from build123d import *

# Parameters (mm, degrees)
F0_W      = 38
F0_H      = 1.8
F1_DEPTH  = 50
F2_W      = 33.097349
F2_H      = 12
F2_W_2    = 36.357001
F3_DEPTH  = 25
F5_W      = 3
F5_H      = 8
F6_DEPTH  = 1.8
F10_R     = 1.2
F11_DEPTH = 43
F4_W      = 33.097349
F4_H      = 12
F4_W_2    = 36.357002
F14_DEPTH = 1


with BuildPart() as f1:
    # F0 (on Top) → F1 (new body)
    with BuildSketch(Plane.XY):
        with Locations((-19, 0)):
            Rectangle(F0_W, F0_H)
        with BuildLine():
            Line((0.167619, 0.9), (0, 0.9))
            Line((0, 0.9), (0, -0.9))
            Line((0, -0.9), (0.167619, -0.9))
            ThreePointArc((0.167619, -0.9), (5, 0), (0.167619, 0.9))
        make_face()
    extrude(amount=F1_DEPTH)

    # F2 (on Right) → F3 (cut)
    with BuildSketch(Plane.YZ):
        with Locations((2.793991, 37)):
            Rectangle(F2_W, F2_H)
        with Locations((3.725327, 13)):
            Rectangle(F2_W_2, F2_H)
    extrude(amount=F3_DEPTH, mode=Mode.SUBTRACT)

    # F5 (on face) → F6 (cut, through all)
    with BuildSketch(Plane.XZ.offset(0.9)):
        with Locations((-32.5, 25)):
            Rectangle(F5_W, F5_H)
        with Locations((-26.5, 25)):
            Rectangle(F5_W, F5_H)
        with Locations((-14.5, 25)):
            Rectangle(F5_W, F5_H)
        with Locations((-8.5, 25)):
            Rectangle(F5_W, F5_H)
    extrude(amount=-F6_DEPTH, mode=Mode.SUBTRACT)

    # F8 (on Front) → F9 (revolve)
    with BuildSketch(Plane.XZ):
        with BuildLine():
            add(Edge.make_bspline(
                [(3.7, 32.2), (3.704607, 31.503535), (3.733649, 31.405747), (4.1, 31)],
                knots=[0, 0, 0, 0, 1.264911, 1.264911, 1.264911, 1.264911], degree=3))
            Line((3.7, 32.2), (2.5, 32.2))
            Line((2.5, 32.2), (2.5, 31))
            Line((2.5, 31), (4.1, 31))
        make_face()
        with BuildLine():
            Line((2.5, 8.2), (2.5, 7))
            Line((2.5, 7), (4.2, 7))
            add(Edge.make_bspline(
                [(4.2, 7), (3.710281, 7), (3.725807, 7.664207), (3.7, 8.2)],
                knots=[0, 0, 0, 0, 1.3, 1.3, 1.3, 1.3], degree=3))
            Line((3.7, 8.2), (2.5, 8.2))
        make_face()
    revolve(axis=Axis((2.5, 0, 31.6), (0, 0, 1)))

    # F10 (on face) → F11 (join, through all)
    with BuildSketch(Plane(origin=(0, 0, 0), x_dir=(1, 0, 0), z_dir=(0, 0, -1))):
        with Locations((2.5, 0)):
            Circle(F10_R)
    extrude(amount=-F11_DEPTH)

    # F12 (on Front) → F13 (revolve)
    with BuildSketch(Plane.XZ):
        with BuildLine():
            Line((4.2, 43), (2.5, 43))
            Line((2.5, 43), (2.5, 41.8))
            Line((2.5, 41.8), (3.7, 41.8))
            add(Edge.make_bspline(
                [(4.2, 43), (3.697237, 42.880607), (3.698886, 42.436921), (3.7, 41.8)],
                knots=[0, 0, 0, 0, 1.3, 1.3, 1.3, 1.3], degree=3))
        make_face()
        with BuildLine():
            Line((4.2, 19), (2.5, 19))
            Line((2.5, 19), (2.5, 17.8))
            Line((2.5, 17.8), (3.7, 17.8))
            add(Edge.make_bspline(
                [(4.2, 19), (3.697237, 18.880607), (3.698886, 18.436921), (3.7, 17.8)],
                knots=[0, 0, 0, 0, 1.3, 1.3, 1.3, 1.3], degree=3))
        make_face()
    revolve(axis=Axis((2.5, 0, 42.4), (0, 0, -1)))

    # F4 (on Right) → F14 (cut)
    with BuildSketch(Plane.YZ):
        with Locations((-0.465668, 37)):
            Rectangle(F4_W, F4_H)
        with Locations((0.465667, 13)):
            Rectangle(F4_W_2, F4_H)
    extrude(amount=-F14_DEPTH, mode=Mode.SUBTRACT)


solid = f1.part
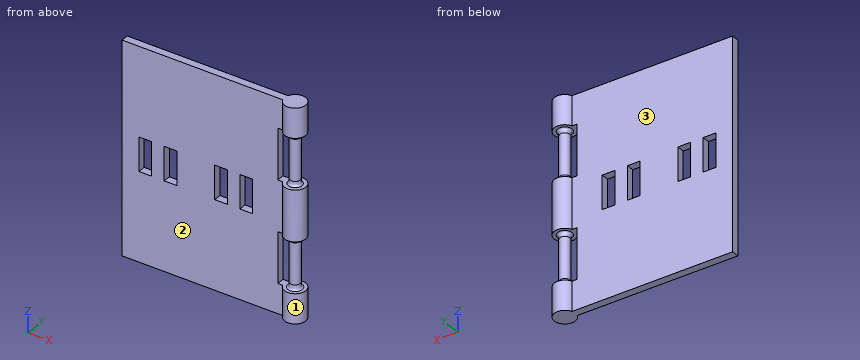
Here's how the part is built. I have some questions about the finished solid (model axes, mm). Face numbers are marked on the shaded views. A direction names the side the tool comes from. Round coordinates to 2 decimals unless told otherwise and drop trailing zeros. Write each loop counter-clockwise with the first axis right and the second up, starting at its lowest first coordinate (ties: lowest second). Pieces come first, ordered by that corner, then holes.
1. For the marked faces 1, 2 and 3, which set-ups out of +Z, -Z, +X, -X, +Y, -Y let a thin tool reach every point of the face, with its end or its side?
2. Suppose I cut it at C-C (x = -24). List the corners of the cut face in (y, z) for me, and give its area (3 significant figures).
3. Suppose I cut it at A-A (z = 35). List the corners of the cut face in (x, y) for me.
4. Will these pins go through, and if not, where does the flat tip stop? pin 1 Ø2 at (x, z) = (-21.5, 41.5) entering from +Y; pin 2 Ø3 at (x, z) = (-14, 29.5) entering from -Y; pin 3 Ø3 at (y, z) = (-1, 33.5) entering from +X.
5. I need wall thicknesses on L1, parallel to Z at x = 0, y = 0.7; L2, parallel to Z at x = -15.5, y = 0.15; L3, parallel to X at y = -0.7, z = 23. Which ranges of each line are inside material? Lowest first, please.
6. Suppose I cut it at B-B (y = 0). State how many separate pieces and enclosed holes the cut face has, and give its area (3 significant figures).
Answer sheet:
1. face 1: +Z, -Z
1. face 2: +Z, -Z, -X, -Y
1. face 3: +Z, -Z, -X, +Y
2. outline: (-0.9, 0) - (0.9, 0) - (0.9, 50) - (-0.9, 50) - close
2. area: 90.0 mm2
3. outline: (-38, -0.9) - (-1, -0.9) - (-1, 0.9) - (-38, 0.9) - close; circle Ø2.4 at (2.5, 0)
4. pin 1: stops at y = 0.9
4. pin 2: stops at y = -0.9
4. pin 3: stops at x = 3.7
5. L1: z = 0 to 7, 19 to 31, 43 to 50
5. L2: z = 0 to 21, 29 to 50
5. L3: x = -38 to -34, -31 to -28, -25 to -16, -13 to -10, -7 to 4.9
6. separate pieces: 1
6. enclosed holes: 6
6. area: 1,970 mm2
